Geometry: see drawing. Coordinates: mm, zero at the bounding-box minimum. Give positions to 0.01 mm unless a question says otherwise; leave off trailing zeros. Order: outer loops, then holes, each group sorted by start corner. A loop starts at its lowest first (then second) coordinate and runs counter-clockwise, first axis right, second up. Notation, with made-up numbers: (59, 86.5) -> (95, 86.5) arc R24 ccw to (95, 111.5) -> close; hole circle Ø2 at (74, 63.25). An arc over 180 degrees is marked (long way). One line per item, written item: value. Start each with the question number.
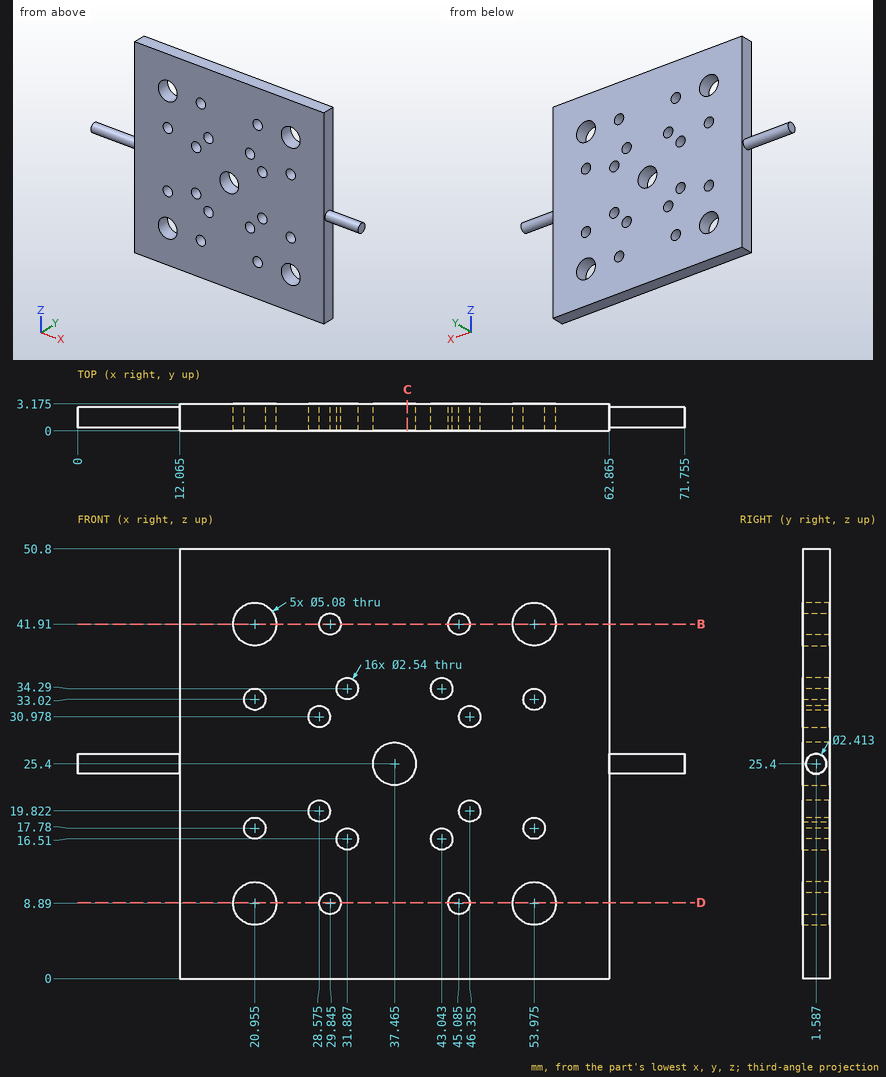
1. Cut plane C-C, the plane x = 39. Return loops of the section in (y, z) (1 decimal).
2. Cut plane B-B, the plane z = 41.91. Return loops of the section in (x, y) (1 decimal).
3. Material intervals for L1, parallel to X at y = 1, z = 41.91 (1 decimal); L2, parallel to Z at x = 30, y = 2.2; L3, parallel to Z at x = 37.5, y = 2.1, sorted ascending. Write a range as [from, to].
4. Cut plane D-D, the plane z = 9. State how many separate pieces and enclosed holes the cut face has, then the cut area to 3 significant figures.
Answers follow:
1. outline: (0, 0) -> (3.2, 0) -> (3.2, 23.4) -> (0, 23.4) -> close; (0, 27.4) -> (3.2, 27.4) -> (3.2, 50.8) -> (0, 50.8) -> close
2. outline: (12.1, 0) -> (18.4, 0) -> (18.4, 3.2) -> (12.1, 3.2) -> close; (23.5, 0) -> (28.6, 0) -> (28.6, 3.2) -> (23.5, 3.2) -> close; (31.1, 0) -> (43.8, 0) -> (43.8, 3.2) -> (31.1, 3.2) -> close; (46.4, 0) -> (51.4, 0) -> (51.4, 3.2) -> (46.4, 3.2) -> close; (56.5, 0) -> (62.9, 0) -> (62.9, 3.2) -> (56.5, 3.2) -> close
3. L1: x = [12.1, 18.4], [23.5, 28.6], [31.1, 43.8], [46.4, 51.4], [56.5, 62.9]
3. L2: z = [0, 7.63], [10.15, 40.65], [43.17, 50.8]
3. L3: z = [0, 22.86], [27.94, 50.8]
4. separate pieces: 5
4. enclosed holes: 0
4. area: 113 mm²
